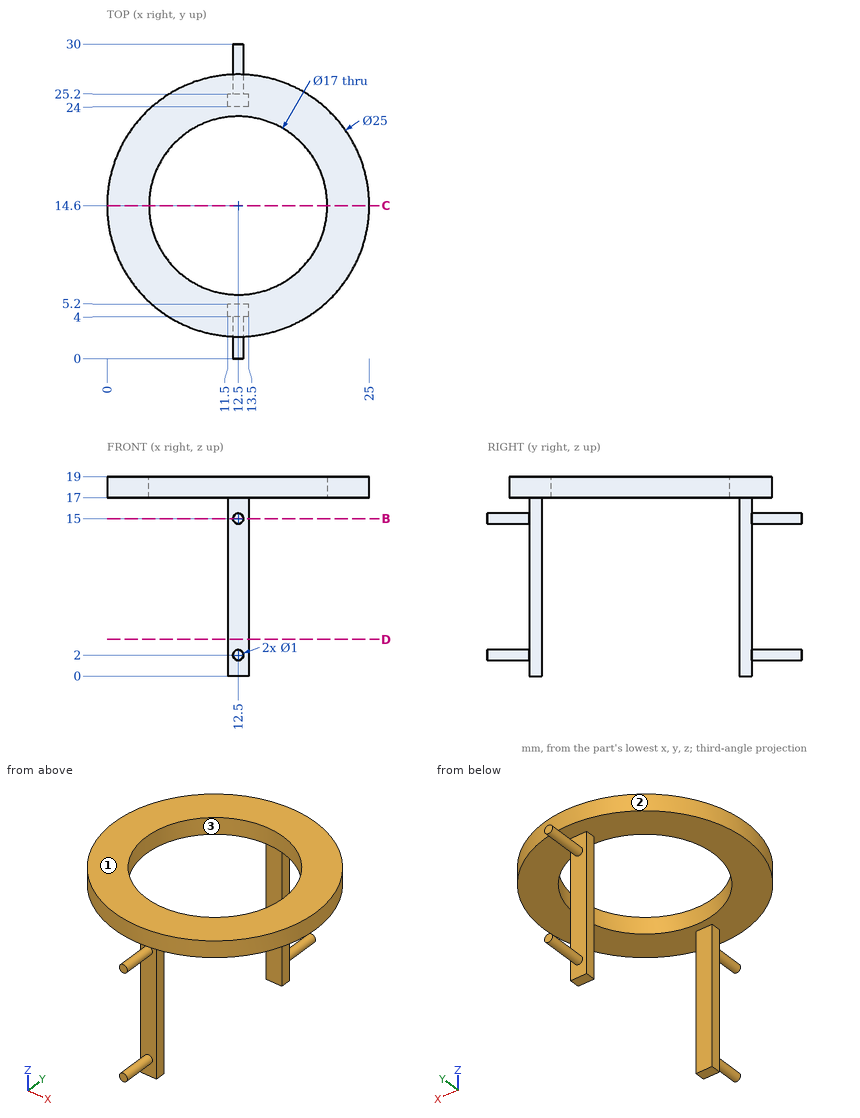
Job drawing, mm, ordinate dimensions from the low corner. One solid piece. Round coordinates to 2 decimals unless told otherwise and drop trailing zeros. Loops run counter-clockwise (first coordinate to the right, second up) from the corner with the lowest first, then second, coordinate; pieces in that order, holes last. Notation, with made-up numbers: M 78,-14.5 L 131,-14.5 A17 ccw 131,17.5 Z; hole C 18,-35 d6. An arc over 180 degrees is marked long. Answer as CSV lines item,"result".
1. Wall check: probe 1 along Y at (x, z) = (12.5, 17.75); probe 2 along Z at (x, y) = (21.25, 17.75); probe 3 along X at (y, z) = (24.25, 9). Give the ranges that are in metal, low to high. Write a range as [from, to].
Resolved:
probe 1,"y = [2.1, 6.1], [23.1, 27.1]"
probe 2,"z = [17, 19]"
probe 3,"x = [11.5, 13.5]"
2. Cut at C-C on y = 14.6. Write the cut outline in (x, z).
Resolved:
outline,"M 0,17 L 4,17 L 4,19 L 0,19 Z; M 21,17 L 25,17 L 25,19 L 21,19 Z"
3. Cut at D-D on z = 3.5. Write the cut outline in (x, y).
Resolved:
outline,"M 11.5,4 L 13.5,4 L 13.5,5.2 L 11.5,5.2 Z; M 11.5,24 L 13.5,24 L 13.5,25.2 L 11.5,25.2 Z"
4. Cut at B-B on z = 15. Write the cut outline in (x, y), then the cut area to 3 significant figures.
Resolved:
outline,"M 11.5,4 L 12,4 L 12,0 L 13,0 L 13,4 L 13.5,4 L 13.5,5.2 L 11.5,5.2 Z; M 11.5,24 L 13.5,24 L 13.5,25.2 L 13,25.2 L 13,30 L 12,30 L 12,25.2 L 11.5,25.2 Z"
area,"13.6 mm²"
5. Flat gauge pins, fed straight in: P1, Ø2, axis at x = 20, y = 11, coming from the -Z side; P2, Ø1, axis at y = 24.5, z = 6, coming from the +X side; P3, Ø1, axis at x = 13, z = 11, coming from the +Y side; P4, Ø4, axis at x = 16, z = 11, coming from the +Y side. Where does each tip first touch, or does it go through?
Resolved:
P1,"stops at z = 17"
P2,"stops at x = 13.5"
P3,"stops at y = 25.2"
P4,"passes through"
6. Two-plate mould, pull along Y, no slides. Class the marked faces 1, 2 and 3: released by +Y, released by -Y, zero draft, split by the parting line, or undercut.
Resolved:
face 1,"zero draft"
face 2,"split by the parting line"
face 3,"undercut"
